Build history of the part. All positions in model axes, mm. A direction names the side the tool comes from. Round coordinates to 2 decimals unless told otherwise and drop trailing zeros. Write each loop counter-clockwise with the first axis right and the second up, starting at its lowest first coordinate (ties: lowest second). Pieces come first, ordered by that corner, then holes.
from build123d import *

# Parameters (mm, degrees)
ESQUISSE1_W             = 300
ESQUISSE1_H             = 70
BOSS_EXTRU_1_DEPTH      = 4
ESQUISSE2_R             = 2.5
ENL_V_MAT_EXTRU_1_DEPTH = 155.081147452
ESQUISSE3_R             = 37.5
ENL_V_MAT_EXTRU_2_DEPTH = 155.081147452
CONG_1_R                = 10
ESQUISSE4_R             = 2
ESQUISSE4_W             = 20
ESQUISSE4_H             = 40
ENL_V_MAT_EXTRU_3_DEPTH = 155.081147452
CONG_2_R                = 5
ESQUISSE5_W             = 10.4
ESQUISSE5_H             = 4.4
ENL_V_MAT_EXTRU_4_DEPTH = 5
ENL_V_MAT_EXTRU_5_DEPTH = 155.081147452


with BuildPart() as part:
    # Esquisse1 → Boss.-Extru.1 (new body)
    with BuildSketch(Plane.XY):
        Rectangle(ESQUISSE1_W, ESQUISSE1_H)
    extrude(amount=BOSS_EXTRU_1_DEPTH)

    # Esquisse2 → Enlèv. mat.-Extru.1 (cut, through all)
    with BuildSketch(Plane.XY.offset(4)):
        with Locations((140, -25)):
            Circle(ESQUISSE2_R)
        with Locations(Location((-140, -25, 0), (0, 0, 180))):
            Circle(ESQUISSE2_R)
        Polygon((-135, -25), (0, -25), (135, -25), (135, -35), (0, -35), (-135, -35), align=None)
    extrude(amount=-ENL_V_MAT_EXTRU_1_DEPTH, mode=Mode.SUBTRACT)

    # Esquisse3 → Enlèv. mat.-Extru.2 (cut, through all)
    with BuildSketch(Plane(origin=(0, 0, 0), x_dir=(-1, 0, 0), z_dir=(0, 0, -1))):
        with Locations((75, 55)):
            Circle(ESQUISSE3_R)
        with Locations((-75, 55)):
            Circle(ESQUISSE3_R)
    extrude(amount=-ENL_V_MAT_EXTRU_2_DEPTH, mode=Mode.SUBTRACT)

    # Congé1
    cong_1_edges = [part.edges().sort_by_distance(p)[0] for p in [
        (-106.721443851, 35, 2),
        (-43.278556149, 35, 2),
        (43.278556149, 35, 2),
        (106.721443851, 35, 2),
    ]]
    fillet(cong_1_edges, radius=CONG_1_R)

    # Esquisse4 → Enlèv. mat.-Extru.3 (cut, through all)
    with BuildSketch(Plane.XY.offset(4)):
        with Locations((-110.9, 30.4)):
            Circle(ESQUISSE4_R)
        with Locations((-121.1, 30.4)):
            Circle(ESQUISSE4_R)
        with Locations((-110.9, -17.4)):
            Circle(ESQUISSE4_R)
        with Locations((-121.1, -17.4)):
            Circle(ESQUISSE4_R)
        with Locations(Location((121.1, -17.4, 0), (0, 0, 180))):
            Circle(ESQUISSE4_R)
        with Locations(Location((110.9, -17.4, 0), (0, 0, 180))):
            Circle(ESQUISSE4_R)
        with Locations(Location((121.1, 30.4, 0), (0, 0, 180))):
            Circle(ESQUISSE4_R)
        with Locations(Location((110.9, 30.4, 0), (0, 0, 180))):
            Circle(ESQUISSE4_R)
        with Locations((-116, 6.5)):
            Rectangle(ESQUISSE4_W, ESQUISSE4_H)
        with Locations((116, 6.5)):
            Rectangle(ESQUISSE4_W, ESQUISSE4_H)
    extrude(amount=-ENL_V_MAT_EXTRU_3_DEPTH, mode=Mode.SUBTRACT)

    # Congé2
    cong_2_edges = [part.edges().sort_by_distance(p)[0] for p in [
        (-135, -25, 2),
        (135, -25, 2),
    ]]
    fillet(cong_2_edges, radius=CONG_2_R)

    # Esquisse5 → Enlèv. mat.-Extru.4 (cut)
    with BuildSketch(Plane(origin=(0, 35, 0), x_dir=(1, 0, 0), z_dir=(0, 1, 0))):
        with Locations((0, -2)):
            Rectangle(ESQUISSE5_W, ESQUISSE5_H)
    extrude(amount=-ENL_V_MAT_EXTRU_4_DEPTH, mode=Mode.SUBTRACT)

    # Esquisse6 → Enlèv. mat.-Extru.5 (cut, through all)
    with BuildSketch(Plane(origin=(0, 0, 0), x_dir=(-1, 0, 0), z_dir=(0, 0, -1))):
        Polygon((-2.1, 30), (2.1, 30), (2.1, 28.2), (3.5, 28.2), (3.5, 25), (2.1, 25), (2.1, 19), (-2.1, 19), (-2.1, 25), (-3.5, 25), (-3.5, 28.2), (-2.1, 28.2), align=None)
    extrude(amount=-ENL_V_MAT_EXTRU_5_DEPTH, mode=Mode.SUBTRACT)


solid = part.part
1) Slice it at A-A (x = -140). Write the cut outline in (y, z).
Results:
outline: (-35, 0) - (-27.5, 0) - (-27.5, 4) - (-35, 4) - close; (-22.5, 0) - (35, 0) - (35, 4) - (-22.5, 4) - close
2) Pin check, flat tips, straight feed: pin 1 Ø1.1 at (x, z) = (2.5, 1) entering from -Y; pin 2 Ø1.5 at (x, z) = (98.5, 1) entering from +Y. Stop position of each tip, or through.
Results:
pin 1: stops at y = -25
pin 2: stops at y = 26.4
3) Wall check: L1, parallel to X at y = 16.5, z = 3.65; L2, parallel to Y at x = 121.1, z = 1.55; L3, parallel to X at y = -31.5, z = 3.05. Give the ranges that are in metal, low to high.
Results:
L1: x = -150 to -126, -106 to 106, 126 to 150
L2: y = -25 to -19.4, -15.4 to -13.5, 26.5 to 28.4, 32.4 to 35
L3: x = -150 to -135, 135 to 150
4) Slice it at D-D (z = 1.75). Count the separate pieces of the cut face and the enclosed holes in it, plus the area to 3 significant figures.
Results:
separate pieces: 1
enclosed holes: 12
area: 14,900 mm2
5) Slice it at C-C (x = -18). Write the cut outline in (y, z).
Results:
outline: (-25, 0) - (35, 0) - (35, 4) - (-25, 4) - close
6) Which spindle directions (+Z, -Z, +X, -X, +Y, -Y) get a long thin tool onto all of the face, cutting with end or side? Do faces 1 (the cylindrical face through (133, -26, 2)), 2 (the flat face through (-2, 0, 4)). Say none if no direction does.
Results:
face 1: +Z, -Z, -Y
face 2: +Z, +X, -X, +Y, -Y
7) Slice it at B-B (y = -3.5). Write the cut outline in (x, z).
Results:
outline: (-150, 0) - (-126, 0) - (-126, 4) - (-150, 4) - close; (-106, 0) - (106, 0) - (106, 4) - (-106, 4) - close; (126, 0) - (150, 0) - (150, 4) - (126, 4) - close
8) Mould opens along X. For faces 3 (the cylindrical face through (-142.385, -25.751, 2.028)), 4 (the flat face through (-2, 0, 0)) say: released by +X, released by -X, zero draft, split by the parting line, or undercut.
Results:
face 3: undercut
face 4: zero draft
